Source: CAD feature listing. Evaluate the final solid. Frame: model axes, mm. Coordinates: 2 decimals unless noted, no trailing zeros. Order: outer loops, then holes, each group sorted by start corner. A loop starts at its lowest first (then second) coordinate and runs counter-clockwise, first axis right, second up.
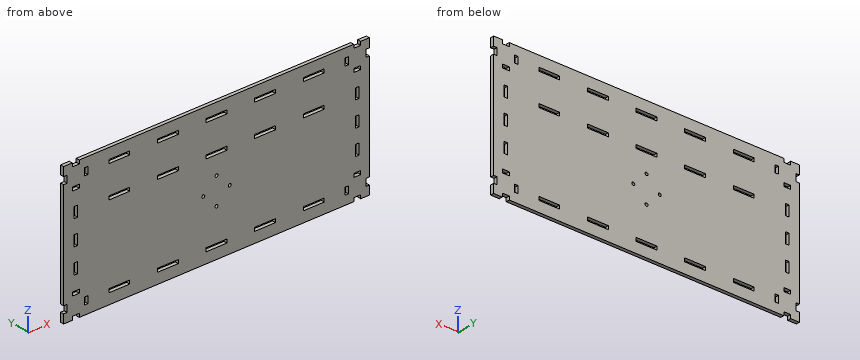
```python
from build123d import *

# Parameters (mm, degrees)
SKETCH2_R           = 2.1
SKETCH2_W           = 30
SKETCH2_H           = 5
SKETCH2_W_2         = 10
SKETCH2_W_3         = 4.999728605
SKETCH2_H_2         = 10
SKETCH2_W_4         = 5
SKETCH2_H_3         = 15
BOSS_EXTRUDE1_DEPTH = 5


with BuildPart() as part:
    # Sketch2 → Boss-Extrude1 (new body)
    with BuildSketch(Plane(origin=(0, -435, 0), x_dir=(1, 0, 0), z_dir=(0, 1, 0))):
        Polygon((-17.5, -95), (-17.5, -100), (-5, -100), (-5, -87.5), (-10, -87.5), (-10, -77.5), (-5, -77.5), (-5, 72.5), (-10, 72.5), (-10, 82.5), (-5, 82.5), (-5, 95), (-17.5, 95), (-17.5, 90), (-27.5, 90), (-27.5, 95), (-422.5, 95), (-422.5, 90), (-432.5, 90), (-432.5, 95), (-445, 95), (-445, 82.5), (-440, 82.5), (-440, 72.5), (-445, 72.5), (-445, -77.5), (-440, -77.5), (-440, -87.5), (-445, -87.5), (-445, -100), (-432.5, -100), (-432.5, -95), (-422.5, -95), (-422.5, -100), (-27.5, -100), (-27.5, -95), align=None)
        with Locations(Location((-225, -9, 0), (0, 0, 270))):
            Circle(SKETCH2_R, mode=Mode.SUBTRACT)
        with Locations(Location((-225, 29, 0), (0, 0, 90))):
            Circle(SKETCH2_R, mode=Mode.SUBTRACT)
        with Locations(Location((-206, 10, 0), (0, 0, 270))):
            Circle(SKETCH2_R, mode=Mode.SUBTRACT)
        with Locations(Location((-244, 10, 0), (0, 0, 90))):
            Circle(SKETCH2_R, mode=Mode.SUBTRACT)
        with Locations((-85, -82.5)):
            Rectangle(SKETCH2_W, SKETCH2_H, mode=Mode.SUBTRACT)
        with Locations((-155, -82.5)):
            Rectangle(SKETCH2_W, SKETCH2_H, mode=Mode.SUBTRACT)
        with Locations((-22.5, 62.5)):
            Rectangle(SKETCH2_W_2, SKETCH2_H, mode=Mode.SUBTRACT)
        with Locations((-225, -82.5)):
            Rectangle(SKETCH2_W, SKETCH2_H, mode=Mode.SUBTRACT)
        with Locations((-37.500135697, 77.5)):
            Rectangle(SKETCH2_W_3, SKETCH2_H_2, mode=Mode.SUBTRACT)
        with Locations((-427.5, -37.5)):
            Rectangle(SKETCH2_W_4, SKETCH2_H_3, mode=Mode.SUBTRACT)
        with Locations((-427.5, 62.5)):
            Rectangle(SKETCH2_W_2, SKETCH2_H, mode=Mode.SUBTRACT)
        with Locations((-427.5, -2.5)):
            Rectangle(SKETCH2_W_4, SKETCH2_H_3, mode=Mode.SUBTRACT)
        with Locations((-412.499864302, 77.5)):
            Rectangle(SKETCH2_W_3, SKETCH2_H_2, mode=Mode.SUBTRACT)
        with Locations((-427.5, 32.5)):
            Rectangle(SKETCH2_W_4, SKETCH2_H_3, mode=Mode.SUBTRACT)
        with Locations((-412.499864302, -82.5)):
            Rectangle(SKETCH2_W_3, SKETCH2_H_2, mode=Mode.SUBTRACT)
        with Locations((-22.5, 32.5)):
            Rectangle(SKETCH2_W_4, SKETCH2_H_3, mode=Mode.SUBTRACT)
        with Locations((-427.5, -67.5)):
            Rectangle(SKETCH2_W_2, SKETCH2_H, mode=Mode.SUBTRACT)
        with Locations((-22.5, -2.5)):
            Rectangle(SKETCH2_W_4, SKETCH2_H_3, mode=Mode.SUBTRACT)
        with Locations((-22.5, -67.5)):
            Rectangle(SKETCH2_W_2, SKETCH2_H, mode=Mode.SUBTRACT)
        with Locations((-22.5, -37.5)):
            Rectangle(SKETCH2_W_4, SKETCH2_H_3, mode=Mode.SUBTRACT)
        with Locations((-37.500135697, -82.5)):
            Rectangle(SKETCH2_W_3, SKETCH2_H_2, mode=Mode.SUBTRACT)
        with Locations((-295, -82.5)):
            Rectangle(SKETCH2_W, SKETCH2_H, mode=Mode.SUBTRACT)
        with Locations((-365, -82.5)):
            Rectangle(SKETCH2_W, SKETCH2_H, mode=Mode.SUBTRACT)
        with Locations((-365, 77.5)):
            Rectangle(SKETCH2_W, SKETCH2_H, mode=Mode.SUBTRACT)
        with Locations((-295, 77.5)):
            Rectangle(SKETCH2_W, SKETCH2_H, mode=Mode.SUBTRACT)
        with Locations((-225, 77.5)):
            Rectangle(SKETCH2_W, SKETCH2_H, mode=Mode.SUBTRACT)
        with Locations((-155, 77.5)):
            Rectangle(SKETCH2_W, SKETCH2_H, mode=Mode.SUBTRACT)
        with Locations((-85, 77.5)):
            Rectangle(SKETCH2_W, SKETCH2_H, mode=Mode.SUBTRACT)
        with Locations((-365, -37.5)):
            Rectangle(SKETCH2_W, SKETCH2_H, mode=Mode.SUBTRACT)
        with Locations((-295, -37.5)):
            Rectangle(SKETCH2_W, SKETCH2_H, mode=Mode.SUBTRACT)
        with Locations((-225, -37.5)):
            Rectangle(SKETCH2_W, SKETCH2_H, mode=Mode.SUBTRACT)
        with Locations((-155, -37.5)):
            Rectangle(SKETCH2_W, SKETCH2_H, mode=Mode.SUBTRACT)
        with Locations((-85, -37.5)):
            Rectangle(SKETCH2_W, SKETCH2_H, mode=Mode.SUBTRACT)
    extrude(amount=BOSS_EXTRUDE1_DEPTH)


solid = part.part
```
1. Section query B-B, the plane y = -433.4. Count the separate pieces of the cut face and the enclosed holes in it, plus the area to 3 significant figures.
2. Contact query for a flat-ended pin moving along its axis: P1, Ø1.5, axis at y = -432, z = 81.5, coming from the -X side. Output: stop coordinate, or through.
3. Section query A-A, the plane x = -359. Output: boundary loops of the cut face in (y, z), plus the area to 3 significant figures.
4. Material intervals for line 1 along X through (y, z) = (-433.35, -39); line 2 along X through (y, z) = (-433.05, -29); line 3 along Z through (x, y) = (-225, -431.45), sorted ascending.
Answer key:
1. separate pieces: 1
1. enclosed holes: 33
1. area: 82,200 mm2
2. P1: stops at x = -440
3. outline: (-435, -95) - (-430, -95) - (-430, -80) - (-435, -80) - close; (-435, -75) - (-430, -75) - (-430, 35) - (-435, 35) - close; (-435, 40) - (-430, 40) - (-430, 80) - (-435, 80) - close; (-435, 85) - (-430, 85) - (-430, 100) - (-435, 100) - close
3. area: 900 mm2
4. line 1: x = -445 to -430, -425 to -25, -20 to -5
4. line 2: x = -445 to -430, -425 to -227.1, -222.9 to -25, -20 to -5
4. line 3: z = -95 to -80, -75 to -31.1, -26.9 to 6.9, 11.1 to 35, 40 to 80, 85 to 100
